Part model, mm, in its own coordinate system. A direction names the side the tool comes from. Round coordinates to 2 decimals unless told otherwise and drop trailing zeros. Order: outer loops, then holes, each group sorted by start corner. A loop starts at its lowest first (then second) coordinate and runs counter-clockwise, first axis right, second up. Notation, with made-up numbers: (65, 49.25) - (98, 49.25) arc R13 ccw to (98, 67.25) - close; hole circle Ø9 at (-11, 44). An arc over 180 degrees is marked (long way). Answer as a JSON object with one key per item and string values.
```python
from build123d import *

# Parameters (mm, degrees)
F0_W     = 30
F0_H     = 20
F1_DEPTH = 20
F2_W     = 5
F2_H     = 10
F3_DEPTH = 20.001
F4_W     = 20
F4_H     = 10
F5_DEPTH = 10
F7_DEPTH = 20.001


with BuildPart() as f1:
    # F0 (on Top) → F1 (new body)
    with BuildSketch(Plane.XY):
        with Locations((15, 10)):
            Rectangle(F0_W, F0_H)
    extrude(amount=F1_DEPTH)

    # F2 (on face) → F3 (cut, through all)
    with BuildSketch(Plane.XY.offset(20)):
        with Locations((27.5, 10)):
            Rectangle(F2_W, F2_H)
    extrude(amount=-F3_DEPTH, mode=Mode.SUBTRACT)

    # F4 (on face) → F5 (cut)
    with BuildSketch(Plane.XY.offset(20)):
        with Locations((10, 10)):
            Rectangle(F4_W, F4_H)
    extrude(amount=-F5_DEPTH, mode=Mode.SUBTRACT)

    # F6 (on face) → F7 (cut, through all)
    with BuildSketch(Plane.XZ):
        Polygon((30, 20), (0, 20), (30, 5), align=None)
    extrude(amount=-F7_DEPTH, mode=Mode.SUBTRACT)


solid = f1.part
```
Item 1: Tool access for faces 1 (the flat face through (30, 2, 2)), 2 (the flat face through (25, 10, 4)), 3 (the flat face through (5, 15, 13)): list every direction of +Z, -Z, +X, -X, +Y, -Y with a clear straight run to the whole face (end or side of a thin tool).
Taken from the geometry:
{"face 1": "+Z, -Z, +X, +Y, -Y", "face 2": "+Z, -Z, +X", "face 3": "+Z, +X, -X"}
Item 2: Cut at D-D (y = 13.5). Write the cut outline in (x, z), plus the area to 3 significant figures.
Taken from the geometry:
{"outline": "(0, 0) - (25, 0) - (25, 7.5) - (20, 10) - (0, 10) - close", "area": "244 mm2"}
Item 3: Two-plate mould, pull along Y, no slides. Class faces 4 (the flat face through (15, 10, 0)), 5 (the flat face through (27, 15, 3)), 6 (the flat face through (11, 20, 8)), 7 (the flat face through (5, 5, 13)): pulls with the +Y half, pulls with the -Y half, needs draft (parallel to the pull), parting line crosses it, or undercut.
Taken from the geometry:
{"face 4": "needs draft", "face 5": "undercut", "face 6": "pulls with the +Y half", "face 7": "undercut"}
Item 4: Probe L1, parallel to Y at x = 9, z = 12; L2, parallel to X at y = 8.5, z = 5.5; L3, parallel to Z at x = 13, y = 12. List the from-to ranges inside material, lowest first. Write a range as from..to.
Taken from the geometry:
{"L1": "0..5, 15..20", "L2": "0..25", "L3": "0..10"}
Item 5: Cut at B-B (x = 3.5). Write the cut outline in (y, z), plus the area to 4 significant figures.
Taken from the geometry:
{"outline": "(0, 0) - (20, 0) - (20, 18.25) - (15, 18.25) - (15, 10) - (5, 10) - (5, 18.25) - (0, 18.25) - close", "area": "282.5 mm2"}
Item 6: Drop flat-ended pins along their axis: P1, Ø3, axis at x = 6.5, y = 10, coming from the +Z side; P2, Ø12, axis at x = 27, z = 18, coming from the -Y side; P3, Ø4, axis at y = 12, z = 2, coming from the +X side; P4, Ø1, axis at x = 8, y = 5, coming from the +Z side. Give the stop position or say it passes through.
Taken from the geometry:
{"P1": "z = 10", "P2": "through", "P3": "x = 25", "P4": "z = 16.25"}
Item 7: Cut at C-C (z = 6.5). Write the cut outline in (x, y).
Taken from the geometry:
{"outline": "(0, 0) - (27, 0) - (27, 5) - (25, 5) - (25, 15) - (27, 15) - (27, 20) - (0, 20) - close"}
Item 8: Cut at A-A (z = 16.75). Write the cut outline in (x, y), plus the area to 3 significant figures.
Taken from the geometry:
{"outline": "(0, 0) - (6.5, 0) - (6.5, 5) - (0, 5) - close; (0, 15) - (6.5, 15) - (6.5, 20) - (0, 20) - close", "area": "65.0 mm2"}
